Can you work these out from the drawing? Everything is in mm from the part's minimum corner. A direction names the side the tool comes from. Coordinates: 2 decimals unless noted, no trailing zeros. Order: outer loops, then holes, each group sorted by start corner. A loop starts at its lowest first (then second) coordinate and runs counter-clockwise, first axis right, second up. Notation, with made-up numbers: (23, -33.75) - (43, -33.75) arc R17 cw to (43, -22.75) - close; hole circle Ø10 at (72.5, 0). An arc over 180 degrees is marked (long way). Answer as CSV lines item,"result". Start each with the question number.
Item 1: Imagine slicing it at A-A on x = 162.5. List the corners of the cut face in (y, z) for me, and give its area (3 significant figures).
Item 2: We'd pull the mould along X, two halves only. Please class the marked faces 3, 4, 5 and 6: pulls with the +X half, pulls with the -X half, needs draft (parallel to the pull), parting line crosses it, or undercut.
Item 3: On a 3-axis mill with a long thin cutter (end or side, diameter ignored), from which of +Z, -Z, +X, -X, +Y, -Y can I reach the whole of each face in a straight line? I mean the marked faces 1 and 2. Say none if no direction works.
Item 4: I need wall thicknesses on line 1 (X direction, y = 3.6, z = 15); line 2 (X direction, y = 41.5, z = 4); line 3 (Y direction, x = 113, z = 26.25). Which ranges of each line are inside material? Lowest first, please.
Item 5: Imagine slicing it at C-C on y = 29.5. List the corners of the cut face in (x, z) for me, and give its area (3 significant figures).
Item 6: I'm going to push a flat-ended pin straight in: pin 1 (4 mm diameter, centred on x = 158, y = 8.5, fed in from -Z). Where does the tip first touch, or does it pass through?
Item 7: Imagine slicing it at B-B on z = 22. List the corners of the cut face in (x, y) for me.
Item 8: Imagine slicing it at D-D on x = 192. List the corners of the cut face in (y, z) for me.
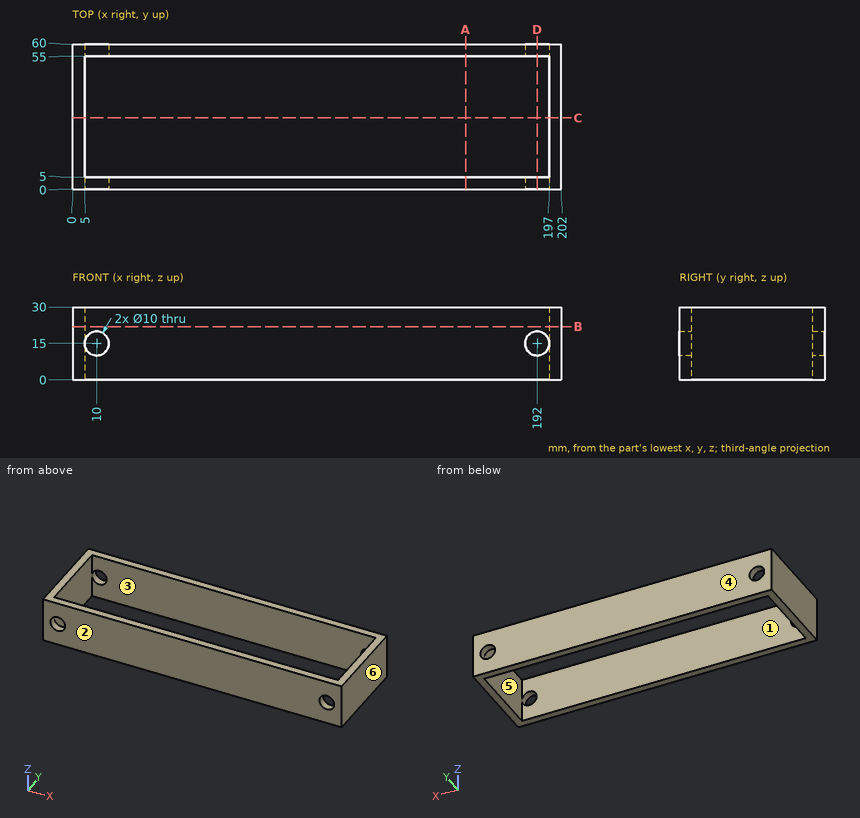
Responses:
1,outline,"(0, 0) - (5, 0) - (5, 30) - (0, 30) - close; (55, 0) - (60, 0) - (60, 30) - (55, 30) - close"
1,area,"300 mm^2"
2,face 3,"undercut"
2,face 4,"needs draft"
2,face 5,"undercut"
2,face 6,"pulls with the +X half"
3,face 1,"+Z, -Z"
3,face 2,"+Z, -Z, +X, -X, -Y"
4,line 1,"x = 0 to 5, 15 to 187, 197 to 202"
4,line 2,"x = 0 to 5, 197 to 202"
4,line 3,"y = 0 to 5, 55 to 60"
5,outline,"(0, 0) - (5, 0) - (5, 30) - (0, 30) - close; (197, 0) - (202, 0) - (202, 30) - (197, 30) - close"
5,area,"300 mm^2"
6,pin 1,"passes through"
7,outline,"(0, 0) - (202, 0) - (202, 60) - (0, 60) - close; hole (5, 5) - (197, 5) - (197, 55) - (5, 55) - close"
8,outline,"(0, 0) - (5, 0) - (5, 10) - (0, 10) - close; (0, 20) - (5, 20) - (5, 30) - (0, 30) - close; (55, 0) - (60, 0) - (60, 10) - (55, 10) - close; (55, 20) - (60, 20) - (60, 30) - (55, 30) - close"
